Design review of the part built by this model. Coordinates are the model's own, in mm. Coordinates: 2 decimals unless noted, no trailing zeros. Loops run counter-clockwise (first coordinate to the right, second up) from the corner with the lowest first, then second, coordinate; pieces in that order, holes last. Notation, with made-up numbers: (39, -8) - (71, -8) arc R10 cw to (71, -1) - close; hole circle Ø3 at (70.5, 0). An arc over 180 degrees is marked (long way). One line per question, with ' | ' between items.
from build123d import *

# Parameters (mm, degrees)
SKIZZE1_R                       = 70
AUFSATZ_LINEAR_AUSTRAGEN1_DEPTH = 20
SKIZZE2_OUTSIDE_W               = 181.8
SKIZZE2_OUTSIDE_H               = 181.8
SKIZZE2_OUTSIDE_R               = 50
SCHNITT_LINEAR_AUSTRAGEN3_DEPTH = 14
SKIZZE3_R                       = 45
SCHNITT_LINEAR_AUSTRAGEN4_DEPTH = 21
VERRUNDUNG1_R                   = 1
FASE1_SIZE                      = 0.5
KREISMUSTER1_COUNT              = 6


with BuildPart() as part:
    # Skizze1 → Aufsatz-Linear austragen1 (new body)
    with BuildSketch(Plane.XY):
        Circle(SKIZZE1_R)
    extrude(amount=AUFSATZ_LINEAR_AUSTRAGEN1_DEPTH)

    # Skizze2 outside → Schnitt-Linear austragen3 (cut)
    with BuildSketch(Plane(origin=(0, 0, 0), x_dir=(-1, 0, 0), z_dir=(0, 0, -1))):
        Rectangle(SKIZZE2_OUTSIDE_W, SKIZZE2_OUTSIDE_H)
        Circle(SKIZZE2_OUTSIDE_R, mode=Mode.SUBTRACT)
    extrude(amount=-SCHNITT_LINEAR_AUSTRAGEN3_DEPTH, mode=Mode.SUBTRACT)

    # Skizze3 → Schnitt-Linear austragen4 (cut, through all)
    with BuildSketch(Plane(origin=(0, 0, 0), x_dir=(-1, 0, 0), z_dir=(0, 0, -1))):
        Circle(SKIZZE3_R)
    extrude(amount=-SCHNITT_LINEAR_AUSTRAGEN4_DEPTH, mode=Mode.SUBTRACT)

    # Verrundung1
    verrundung1_edges = [part.edges().sort_by_distance(p)[0] for p in [
        (50, 0, 14),
    ]]
    fillet(verrundung1_edges, radius=VERRUNDUNG1_R)

    # Fase1
    fase1_edges = [part.edges().sort_by_distance(p)[0] for p in [
        (-70, 0, 14),
    ]]
    chamfer(fase1_edges, length=FASE1_SIZE)

    # Skizze8 → M2 Gewindebohrung1 (revolve, cut)
    with BuildSketch(Plane(origin=(-47.5, -4.651151255, 0), x_dir=(0, 1, 0), z_dir=(1, 0, 0))):
        Polygon((0, 0), (0, 10.480688495), (0.8, 10), (0.8, 0), align=None)
    m2_gewindebohrung1 = revolve(axis=Axis((-47.5, -4.651151255, -6.35), (0, 0, 1)), mode=Mode.SUBTRACT)

    # Kreismuster1: M2 Gewindebohrung1 ×6 about axis
    kreismuster1_axis = Axis((0, 0, 0), (0, 0, 1))
    for i in range(1, KREISMUSTER1_COUNT):
        add(m2_gewindebohrung1.rotate(kreismuster1_axis, i * 360 / KREISMUSTER1_COUNT), mode=Mode.SUBTRACT)


solid = part.part
Q1. Take a section at A-A (x = 0). Give the boundary of the cut face in (y, z), plus the area to 3 significant figures.
Returned:
outline: (-70, 14.5) - (-69.5, 14) - (-51, 14) arc R1 cw to (-50, 13) - (-50, 0) - (-45, 0) - (-45, 20) - (-70, 20) - close; (45, 0) - (50, 0) - (50, 13) arc R1 cw to (51, 14) - (69.5, 14) - (70, 14.5) - (70, 20) - (45, 20) - close | area: 440 mm²
Q2. Take a section at D-D (z = 16.75). Give the boundary of the cut face in (x, y).
Returned:
outline: circle Ø140 at (0, 0); hole circle Ø90 at (0, 0)
Q3. To check wall thickness, follow line 1 along X through (y, z) = (0.5, 4); line 2 along X through (y, z) = (4, 9.5); line 3 along Z through (x, y) = (3.5, -51). State the ranges of each line that lie inside material, in increasing order.
Returned:
line 1: x = -50 to -45, 45 to 50 | line 2: x = -49.84 to -44.82, 44.82 to 47.04, 47.96 to 49.84 | line 3: z = 14 to 20
Q4. For pin 1 (6 mm diameter, centred on y = 25, z = 6.5, fed in from -X); pin 2 (12 mm diameter, centred on x = 48.5, z = 7, fed in from +Y); pin 3 (3 mm diameter, centred on x = 26, y = -47, fed in from -Z), all flat-tipped, find the tip position at first contact; note any pin that passes through.
Returned:
pin 1: stops at x = -44.9 | pin 2: stops at y = 26.34 | pin 3: stops at z = 14
Q5. Draft analysis for pull direction X (two halves, no side actions). For faces 1 (the flat face through (21, 47, 14)), 2 (the cylindrical face through (-20.765, -39.923, 9.86)), 3 (the cylindrical face through (-47.69, 15.02, 6.41)), state which applies: +X half, -X half, draft (parallel to the pull), parting line (faces both ways), or undercut.
Returned:
face 1: draft | face 2: undercut | face 3: parting line
Q6. Take a section at C-C (z = 7.5). Give the boundary of the cut face in (x, y), plus the area to 3 significant figures.
Returned:
outline: circle Ø100 at (0, 0); hole circle Ø1.6 at (-47.5, -4.65); hole circle Ø90 at (0, 0); hole circle Ø1.6 at (-27.78, 38.81); hole circle Ø1.6 at (-19.72, -43.46); hole circle Ø1.6 at (19.72, 43.46); hole circle Ø1.6 at (27.78, -38.81); hole circle Ø1.6 at (47.5, 4.65) | area: 1,480 mm²
